```python
from build123d import *

# Parameters (mm, degrees)
SKETCH1_R           = 1.5
SKETCH1_R_2         = 11.5
SKETCH1_R_3         = 2.495506105
BOSS_EXTRUDE1_DEPTH = 33
SKETCH1_3_R         = 11.5
BOSS_EXTRUDE2_DEPTH = 35
SKETCH1_4_R         = 2.495506105
BOSS_EXTRUDE3_DEPTH = 57
SKETCH1_5_W         = 5.430918786
SKETCH1_5_H         = 16.000755457
BOSS_EXTRUDE4_DEPTH = 7


with BuildPart() as part:
    # Sketch1 → Boss-Extrude1 (new body)
    # profile 1 of 3: a face of its own
    with BuildSketch(Plane.XY):
        Polygon((-15.184651762, 21.5), (-18.505405032, 18.179246731), (-18.505405032, 8.037627152), (-18.505405032, -7.963128305), (-18.505405032, -18.179246731), (-15.184651762, -21.5), (20.470167461, -21.5), (24.494594968, -19.079506704), (24.494594968, 18.915642106), (20.57338357, 21.5), align=None)
        with Locations((-12.211230799, -15.205825767)):
            Circle(SKETCH1_R, mode=Mode.SUBTRACT)
        with Locations((18.200420735, -15.205825767)):
            Circle(SKETCH1_R, mode=Mode.SUBTRACT)
        with Locations((-12.211230799, 15.205825767)):
            Circle(SKETCH1_R, mode=Mode.SUBTRACT)
        with Locations((2.994594968, 0)):
            Circle(SKETCH1_R_2, mode=Mode.SUBTRACT)
        with Locations((18.200420735, 15.205825767)):
            Circle(SKETCH1_R, mode=Mode.SUBTRACT)
    # profile 2 of 3: a face of its own
    with BuildSketch(Plane.XY):
        with Locations((2.994594968, 0)):
            Circle(SKETCH1_R_2)
        with Locations((2.994594968, 0)):
            Circle(SKETCH1_R_3, mode=Mode.SUBTRACT)
    # profile 3 of 3: a face of its own
    with BuildSketch(Plane.XY):
        with Locations((2.994594968, 0)):
            Circle(SKETCH1_R_3)
    extrude(amount=BOSS_EXTRUDE1_DEPTH)

    # Sketch1_3 → Boss-Extrude2 (add)
    with BuildSketch(Plane.XY):
        with Locations((2.994594968, 0)):
            Circle(SKETCH1_3_R)
    extrude(amount=BOSS_EXTRUDE2_DEPTH)

    # Sketch1_4 → Boss-Extrude3 (add)
    with BuildSketch(Plane.XY):
        with Locations((2.994594968, 0)):
            Circle(SKETCH1_4_R)
    extrude(amount=BOSS_EXTRUDE3_DEPTH)

    # Sketch1_5 → Boss-Extrude4 (add)
    with BuildSketch(Plane.XY):
        with Locations((-21.220864425, 0.037249424)):
            Rectangle(SKETCH1_5_W, SKETCH1_5_H)
    extrude(amount=BOSS_EXTRUDE4_DEPTH)


solid = part.part
```
Can you work these out from the model? Positions are in its coordinate system, mm. A direction names the side the tool comes from. Give positions to 0.01 mm unless a question says otherwise; leave off trailing zeros. Loops run counter-clockwise (first coordinate to the right, second up) from the corner with the lowest first, then second, coordinate; pieces in that order, holes last. Notation, with made-up numbers: M 56.25,37 L 81.25,37 A13 cw 81.25,48 Z; hole C -14.75,55.25 d10. An arc over 180 degrees is marked long. One line per item, written item: value.
(1) Suppose I cut it at B-B on z = 12.5. List the corners of the cut face in (x, y) for me.
Returned:
outline: M -18.51,-18.18 L -15.18,-21.5 L 20.47,-21.5 L 24.49,-19.08 L 24.49,18.92 L 20.57,21.5 L -15.18,21.5 L -18.51,18.18 Z; hole C -12.21,-15.21 d3; hole C -12.21,15.21 d3; hole C 18.2,-15.21 d3; hole C 18.2,15.21 d3
(2) Suppose I cut it at A-A on y = -3.5. List the corners of the cut face in (x, z) for me.
Returned:
outline: M -23.94,0 L 24.49,0 L 24.49,33 L 13.95,33 L 13.95,35 L -7.96,35 L -7.96,33 L -18.51,33 L -18.51,7 L -23.94,7 Z
(3) Which directions (+Z, -Z, +X, -X, +Y, -Y) give clear straight access to the entire face, cutting with the end or side of a thin tool? Please do faces 1 (the face through (-21, -7.963, 3)), 2 (the face through (-21, 8.038, 3)), 3 (the face through (19.63, 15.66, 16.27)), 4 (the face through (2.67, 2.474, 45.846)).
Returned:
face 1: +Z, -Z, -X, -Y
face 2: +Z, -Z, -X, +Y
face 3: +Z, -Z
face 4: +Z
(4) Will these pins go through, and if not, where does the flat tip stop? pin 1 (12 mm diameter, centred on y = 16.5, z = 33, fed in from -X); pin 2 (5 mm diameter, centred on x = 4.5, z = 36.5, fed in from +Y); pin 3 (5 mm diameter, centred on x = 18.2, y = 15.21, fed in from -Z); pin 4 (4 mm diameter, centred on x = -12.21, y = -15.21, fed in from +Z).
Returned:
pin 1: x = -18.51
pin 2: y = 11.5
pin 3: z = 0
pin 4: z = 33
(5) Suppose I cut it at D-D on z = 37.5. List the corners of the cut face in (x, y) for me.
Returned:
outline: C 2.99,0 d4.99
(6) We'd pull the mould along X, two halves only. Please class faces 5 (the face through (-16.822, 19.863, 16.269)), 6 (the face through (22.56, 20.19, 16.27)), 7 (the face through (-11.405, -13.941, 16.269)): released by +X, released by -X, zero draft, split by the parting line, or undercut.
Returned:
face 5: released by -X
face 6: released by +X
face 7: undercut
(7) Suppose I cut it at C-C on x = -3.5. List the corners of the cut face in (y, z) for me, plus the area to 3 significant figures.
Returned:
outline: M -21.5,0 L 21.5,0 L 21.5,33 L 9.49,33 L 9.49,35 L -9.49,35 L -9.49,33 L -21.5,33 Z
area: 1,460 mm^2
(8) I need wall thicknesses on line 1 (Z direction, x = 15.5, y = -17); line 2 (X direction, y = 17, z = 14); line 3 (Z direction, x = -20, y = 5.5). Which ranges of each line are inside material? Lowest first, please.
Returned:
line 1: 0 to 33
line 2: -18.51 to 24.49
line 3: 0 to 7
